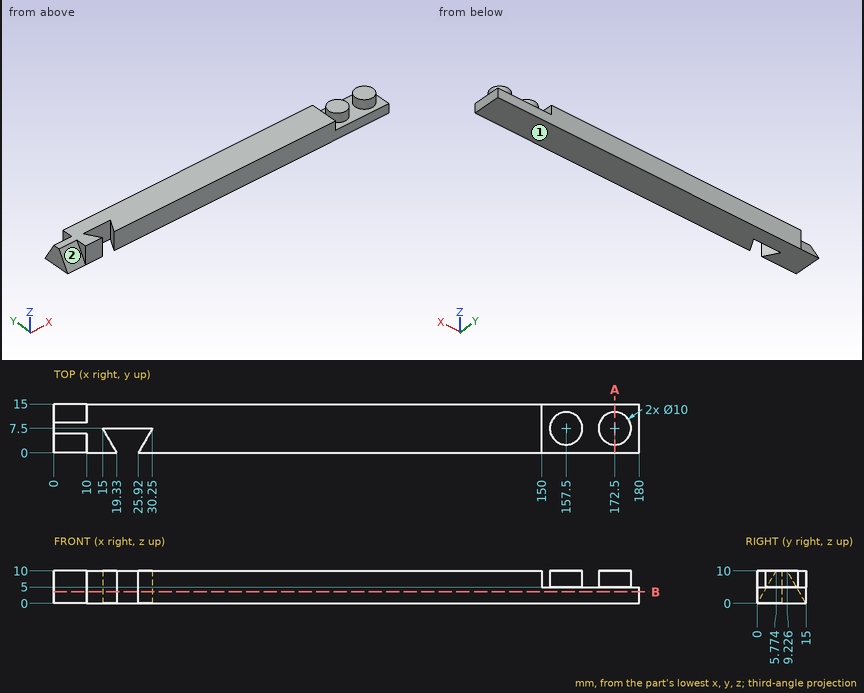
Part print with two shaded views. Sizes in mm from the minimum x, y, z corner. A direction names the side the tool comes from. Coordinates: 2 decimals unless noted, no trailing zeros. Order: outer loops, then holes, each group sorted by start corner. A loop starts at its lowest first (then second) coordinate and runs counter-clockwise, first axis right, second up. Notation, with made-up numbers: (-11.75, 87) - (17.25, 87) arc R26 ccw to (17.25, 101) - close; hole circle Ø4 at (-16, 69). An arc over 180 degrees is marked (long way). Write item = value, one per line. Start each with the question number.
1) Wall check: line 1 along X through (y, z) = (4.5, 9.25); line 2 along X through (y, z) = (10.5, 6.5); line 3 along X through (y, z) = (8.5, 7). Give the ranges that are in metal, low to high. Write a range as from..to.
2) Saw through at A-A on x = 172.5. Write the cut outline in (y, z).
3) 3-axis set-ups, long thin cutter, end or side, ignore diameter. For the marked faces 1 and 2: which of +Z, -Z, +X, -X, +Y, -Y reach the whole face in a straight line?
4) Saw through at B-B on z = 3.5. Write the cut outline in (x, y), then the cut area to 3 significant figures.
5) Flat gauge pins, fed straight in: pin 1 Ø1 at (x, z) = (22, 6) entering from -Y; pin 2 Ø3 at (y, z) = (13, 7) entering from -X; pin 3 Ø4 at (y, z) = (6, 7.5) entering from +X. Where does each tip first touch, or does it go through?
From the geometry:
q1.line_1 = 10..16.73, 28.52..150, 153.5..161.5, 168.5..176.5
q1.line_2 = 0..150, 153.5..161.5, 168.5..176.5
q1.line_3 = 0..150, 152.6..162.4, 167.6..177.4
q2.outline = (0, 0) - (15, 0) - (15, 5) - (12.5, 5) - (12.5, 10) - (2.5, 10) - (2.5, 5) - (0, 5) - close
q3.face_1 = -Z, +X, -X, +Y, -Y
q3.face_2 = +Z, -X, -Y
q4.outline = (0, 2.02) - (10, 2.02) - (10, 0) - (19.33, 0) - (15, 7.5) - (30.25, 7.5) - (25.92, 0) - (180, 0) - (180, 15) - (10, 15) - (10, 12.98) - (0, 12.98) - close
q4.area = 2,580 mm^2
q5.pin_1 = 7.5
q5.pin_2 = 10
q5.pin_3 = 177.5
